from build123d import *

# Parameters (mm, degrees)
CROQUIS1_W              = 17
CROQUIS1_H              = 15
SALIENTE_EXTRUIR1_DEPTH = 12.5
CROQUIS2_R              = 2.75
CORTAR_EXTRUIR1_DEPTH   = 20
CROQUIS4_R              = 1.5
CORTAR_EXTRUIR3_DEPTH   = 20
CROQUIS8_W              = 15
CROQUIS8_H              = 3
SALIENTE_EXTRUIR2_DEPTH = 10
CROQUIS9_R              = 1.5
CORTAR_EXTRUIR6_DEPTH   = 6
CROQUIS10_W             = 3
CROQUIS10_H             = 15
SALIENTE_EXTRUIR3_DEPTH = 8
CROQUIS11_R             = 1.5
CORTAR_EXTRUIR8_DEPTH   = 6


with BuildPart() as part:
    # Croquis1 → Saliente-Extruir1 (new body)
    with BuildSketch(Plane(origin=(0, 0, 0), x_dir=(1, 0, 0), z_dir=(0, 1, 0))):
        Rectangle(CROQUIS1_W, CROQUIS1_H)
    extrude(amount=SALIENTE_EXTRUIR1_DEPTH)

    # Croquis2 → Cortar-Extruir1 (cut)
    with BuildSketch(Plane(origin=(0, 0, -7.5), x_dir=(-1, 0, 0), z_dir=(0, 0, -1))):
        with Locations((0, 7.5)):
            Circle(CROQUIS2_R)
        with BuildLine():
            Line((0.5, 12.5), (-0.5, 12.5))
            Line((-0.5, 12.5), (-0.5, 10.204163457))
            ThreePointArc((-0.5, 10.204163457), (0, 10.25), (0.5, 10.204163457))
            Line((0.5, 10.204163457), (0.5, 12.5))
        make_face()
    extrude(amount=-CORTAR_EXTRUIR1_DEPTH, mode=Mode.SUBTRACT)

    # Croquis4 → Cortar-Extruir3 (cut)
    with BuildSketch(Plane.ZY.offset(8.5)):
        with Locations((-0.5, 7.5)):
            Circle(CROQUIS4_R)
    extrude(amount=-CORTAR_EXTRUIR3_DEPTH, mode=Mode.SUBTRACT)

    # Croquis8 → Saliente-Extruir2 (add)
    with BuildSketch(Plane.ZY.offset(8.5)):
        with Locations((0, 1.5)):
            Rectangle(CROQUIS8_W, CROQUIS8_H)
    extrude(amount=SALIENTE_EXTRUIR2_DEPTH)

    # Croquis9 → Cortar-Extruir6 (cut)
    with BuildSketch(Plane(origin=(0, 3, 0), x_dir=(1, 0, 0), z_dir=(0, 1, 0))):
        with Locations((-13.5, 0)):
            Circle(CROQUIS9_R)
    extrude(amount=-CORTAR_EXTRUIR6_DEPTH, mode=Mode.SUBTRACT)

    # Croquis10 → Saliente-Extruir3 (add)
    with BuildSketch(Plane(origin=(0, 12.5, 0), x_dir=(1, 0, 0), z_dir=(0, 1, 0))):
        with Locations((7, 0)):
            Rectangle(CROQUIS10_W, CROQUIS10_H)
    extrude(amount=SALIENTE_EXTRUIR3_DEPTH)

    # Croquis11 → Cortar-Extruir8 (cut)
    with BuildSketch(Plane.ZY.offset(-5.5)):
        with Locations((3.5, 16.5)):
            Circle(CROQUIS11_R)
        with Locations((-3.5, 16.5)):
            Circle(CROQUIS11_R)
    extrude(amount=-CORTAR_EXTRUIR8_DEPTH, mode=Mode.SUBTRACT)


solid = part.part
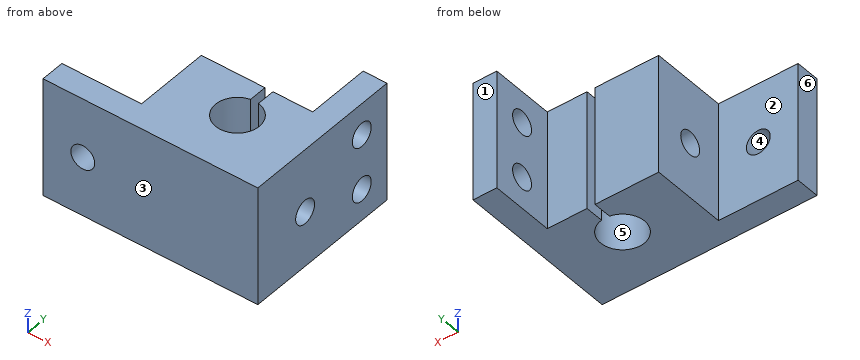
Check sheet for the modelled part. Datum: model origin and axes. Units: mm. Face numbers are marked on the shaded views. A direction names the side the tool comes from. Coordinates: 2 decimals unless noted, no trailing zeros. Write each loop counter-clockwise with the first axis right and the second up, starting at its lowest first coordinate (ties: lowest second). Pieces come first, ordered by that corner, then holes.
Item 1: Cross-section at A-A on y = 16.5. Record the boundary of the cut face in (x, z), then the cut area to 3 significant figures.
Numbers:
outline: (5.5, -7.5) - (8.5, -7.5) - (8.5, -5) - (5.5, -5) - close; (5.5, -2) - (8.5, -2) - (8.5, 2) - (5.5, 2) - close; (5.5, 5) - (8.5, 5) - (8.5, 7.5) - (5.5, 7.5) - close
area: 27.0 mm2
Item 2: Scan lines: probe 1 along X at (y, z) = (7.5, 3); probe 2 along X at (y, z) = (10.5, -3.5); probe 3 along Y at (x, z) = (7.3, -3.5). Record each from-to range of solid material in increasing order.
Numbers:
probe 1: x = -8.5 to -2.75, 2.75 to 8.5
probe 2: x = -8.5 to -0.5, 0.5 to 8.5
probe 3: y = 0 to 15, 18 to 20.5
Item 3: Mould release check, pull along X, two halves, no side actions. Record for the marked faces 3, 4, 5 and 6: released by +X, released by -X, zero draft, split by the parting line, or undercut.
Numbers:
face 3: zero draft
face 4: undercut
face 5: undercut
face 6: released by -X
Item 4: Cross-section at D-D on y = 12. Record the boundary of the cut face in (x, z), then the cut area to 3 significant figures.
Numbers:
outline: (-8.5, -7.5) - (-0.5, -7.5) - (-0.5, 7.5) - (-8.5, 7.5) - close; (0.5, -7.5) - (8.5, -7.5) - (8.5, 7.5) - (0.5, 7.5) - close
area: 240 mm2
Item 5: Cross-section at B-B on z = 3.5. Record the boundary of the cut face in (x, y).
Numbers:
outline: (-18.5, 0) - (8.5, 0) - (8.5, 15) - (5.5, 15) - (5.5, 12.5) - (0.5, 12.5) - (0.5, 10.2) arc R2.75 cw (long way) to (-0.5, 10.2) - (-0.5, 12.5) - (-8.5, 12.5) - (-8.5, 3) - (-18.5, 3) - close; (5.5, 18) - (8.5, 18) - (8.5, 20.5) - (5.5, 20.5) - close
Item 6: Access from +Z, -Z, +X, -X, +Y, -Y to the whole of each face (thin tool, end or side, straight path). Record for the marked faces 1 and 2.
Numbers:
face 1: +Z, -Z, +X, -X, +Y
face 2: +Z, -Z, -X, +Y
Item 7: Cross-section at C-C on x = -13.5. Record the boundary of the cut face in (y, z).
Numbers:
outline: (0, -7.5) - (3, -7.5) - (3, -1.5) - (0, -1.5) - close; (0, 1.5) - (3, 1.5) - (3, 7.5) - (0, 7.5) - close
Item 8: Depth check by flat-ended pin: pin 1 Ø2.5 at (x, z) = (-4.5, -3.5) entering from +Y; pin 2 Ø1 at (y, z) = (5, 2) entering from -X; pin 3 Ø6 at (x, y) = (-13, 13) entering from +Z; pin 4 Ø2 at (x, z) = (-12, -4) entering from +Y. Enter the tip coordinate at first touch or a pass-through.
Numbers:
pin 1: stops at y = 12.5
pin 2: stops at x = -8.5
pin 3: passes through
pin 4: stops at y = 3
